from build123d import *

# Parameters (mm, degrees)
SKETCH_1_W                                   = 1050
SKETCH_1_H                                   = 800
PAD001_DEPTH                                 = 21
SKETCH003_R                                  = 4
SKETCH003_R_2                                = 2
POCKET_DEPTH                                 = 0.001
POCKET_DEPTH_BACK                            = 21.001
POCKET001_DEPTH                              = 0.001
POCKET001_DEPTH_BACK                         = 21.001
PLYWOOD_CUTTING_ROLL_SUPPORT_PLACEMENT_ANGLE = 180


with BuildPart() as part:
    # Sketch_1 → Pad001 (new body)
    with BuildSketch(Plane.XY):
        with Locations((25, -100)):
            Rectangle(SKETCH_1_W, SKETCH_1_H)
    extrude(amount=PAD001_DEPTH)

    # Sketch003 → Pocket (cut, two sides)
    with BuildSketch(Plane.XY) as pocket_sk:
        with Locations((-398.3, -47.5)):
            Circle(SKETCH003_R)
        with Locations((-398.3, 47.5)):
            Circle(SKETCH003_R)
        with Locations((398.3, -47.5)):
            Circle(SKETCH003_R)
        with Locations((398.3, 47.5)):
            Circle(SKETCH003_R)
        with Locations((-437.9, -147.5)):
            Circle(SKETCH003_R)
        with Locations((-437.9, -52.5)):
            Circle(SKETCH003_R)
        with Locations((437.9, -147.5)):
            Circle(SKETCH003_R)
        with Locations((437.9, -52.5)):
            Circle(SKETCH003_R)
        with Locations((15, -140)):
            Circle(SKETCH003_R_2)
        with Locations((15, -60)):
            Circle(SKETCH003_R_2)
        with Locations((315, -60)):
            Circle(SKETCH003_R_2)
        with Locations((315, -140)):
            Circle(SKETCH003_R_2)
        with Locations((-285, -140)):
            Circle(SKETCH003_R_2)
        with Locations((-285, -60)):
            Circle(SKETCH003_R_2)
        with Locations((-418, -252.5)):
            Circle(SKETCH003_R_2)
        with Locations((-418, -347.5)):
            Circle(SKETCH003_R_2)
        with Locations((0, -203)):
            Circle(SKETCH003_R_2)
        with Locations((333.333333, -203)):
            Circle(SKETCH003_R_2)
        with Locations((-333.333333, -203)):
            Circle(SKETCH003_R_2)
    extrude(amount=-POCKET_DEPTH, mode=Mode.SUBTRACT)
    extrude(pocket_sk.sketch, amount=POCKET_DEPTH_BACK, mode=Mode.SUBTRACT)

    # Sketch008 → Pocket001 (cut, two sides)
    with BuildSketch(Plane.XY) as pocket001_sk:
        Polygon((-417.3, 63.5), (-417.3, -36.480682), (-456.873413, -36.480682), (-456.873413, -163.480682), (-754.283264, -163.480682), (-754.283264, 63.5), align=None)
    extrude(amount=-POCKET001_DEPTH, mode=Mode.SUBTRACT)
    extrude(pocket001_sk.sketch, amount=POCKET001_DEPTH_BACK, mode=Mode.SUBTRACT)


with BuildPart() as part_1:
    # plywood_cutting_roll_support placement: moved
    add(part.part.moved(Location((0, 65, 0))).rotate(Axis((0, 65, 0), (0, 0, 1)), PLYWOOD_CUTTING_ROLL_SUPPORT_PLACEMENT_ANGLE))


solid = part_1.part
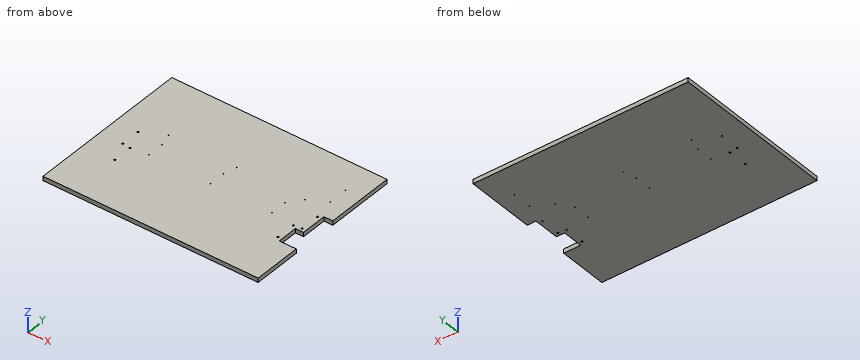
CAD build for the part. Positions are in the model's coordinates, mm. Give positions to 0.01 mm unless a question says otherwise; leave off trailing zeros. Put each result on its own line as item: value. Start each with the question number.
(1) Band-saw the part on A-A, the plane z = 3.25. Give the number of separate pieces and of enclosed holes in the cut face, and give its area (3 significant figures).
(2) Flat gauge pins, fed straight in: pin 1 Ø4.5 at (x, y) = (285, 125) entering from -Z; pin 2 Ø3 at (y, z) = (197, 4.5) entering from +X; pin 3 Ø3 at (x, y) = (-315, 125) entering from +Z; pin 4 Ø6.5 at (y, z) = (60, 6) entering from +X. Where does each tip first touch, or does it go through?
(3) Probe L1, parallel to Y at x = -437.9, z = 14; L2, parallel to Y at x = -398.3, z = 4.5; L3, parallel to Y at x = 437.9, z = 12. List the from-to ranges inside material, lowest first.
Response values:
1. separate pieces: 1
1. enclosed holes: 19
1. area: 826,000 mm2
2. pin 1: stops at z = 0
2. pin 2: stops at x = 456.87
2. pin 3: passes through
2. pin 4: stops at x = 417.3
3. L1: y = -235 to 113.5, 121.5 to 208.5, 216.5 to 565
3. L2: y = -235 to 13.5, 21.5 to 108.5, 116.5 to 565
3. L3: y = -235 to 1.5, 101.48 to 113.5, 121.5 to 208.5, 216.5 to 565
